from build123d import *

# Parameters (mm, degrees)
F1_DEPTH = 24
F5_R     = 5.08


with BuildPart() as f1:
    # F0 (on Top) → F1 (new body)
    with BuildSketch(Plane.XY):
        with BuildLine():
            Line((-131, 0), (0, 0))
            Line((0, 0), (0, 762))
            Line((0, 762), (-643, 762))
            ThreePointArc((-643, 762), (-996.5533905933, 615.5533905933), (-1143, 262))
            Line((-1143, 262), (-1143, -381))
            Line((-1143, -381), (-381, -381))
            Line((-381, -381), (-381, -250))
            ThreePointArc((-381, -250), (-307.7766952966, -73.2233047034), (-131, 0))
        make_face()
    extrude(amount=F1_DEPTH)

    # F4: sweep along a path in F3
    with BuildLine(Plane(origin=(0, 0, 0), x_dir=(1, 0, 0), z_dir=(0, 0, -1))) as f4_path:
        Line((-381, 381), (-1143, 381))
        Line((-1143, 381), (-1143, -262))
        ThreePointArc((-1143, -262), (-996.5533905933, -615.5533905933), (-643, -762))
        Line((-643, -762), (0, -762))
        Line((0, -762), (0, 0))
        Line((0, 0), (-131, 0))
        ThreePointArc((-131, 0), (-307.7766952966, 73.2233047034), (-381, 250))
        Line((-381, 250), (-381, 381))
    # F2 (on face) → F4 (sweep, cut)
    with BuildSketch(Plane.YZ):
        Polygon((762, 0), (762, 14), (712, 0), align=None)
    sweep(path=f4_path.line, transition=Transition.RIGHT, mode=Mode.SUBTRACT)

    # F5
    f5_edges = [f1.edges().sort_by_distance(p)[0] for p in [
        (0, 762, 19),
        (0, 0, 19),
        (-381, -381, 19),
        (-1143, -381, 19),
    ]]
    fillet(f5_edges, radius=F5_R)


solid = f1.part
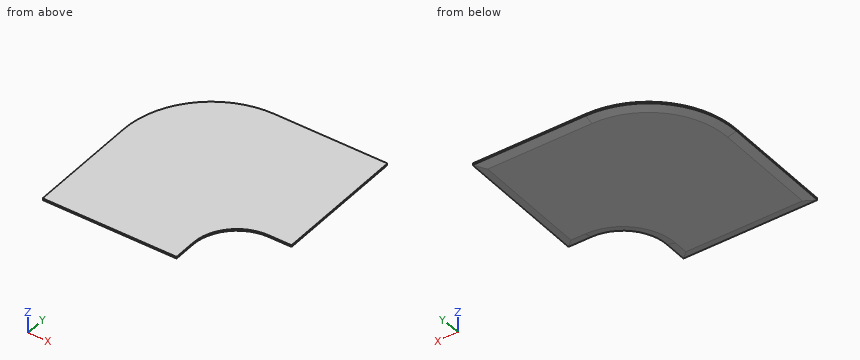
Input: part model. Units: mm. Frame: model coordinates. Coordinates: 2 decimals unless noted, no trailing zeros. Loops run counter-clockwise (first coordinate to the right, second up) from the corner with the lowest first, then second, coordinate; pieces in that order, holes last.
(1) Section B-B on y = 218.5. Return the cut outline in (x, z).
(2) Section A-A on z = 18.25. Return the cut outline in (x, y).
(3) Material intervals for probe 1 along Y at (x, z) = (-71, 20); probe 2 along Y at (x, z) = (-722, 18.25), sorted ascending.
(4) First-contact query: pin 1 Ø1 at (x, y) = (-285, -53.5) entering from -Z; pin 2 Ø5 at (y, z) = (-319, 19) entering from +X; pin 3 Ø5 at (x, z) = (-77.5, 17) entering from -Y. Flat tips, straight axial feed; report the tip coordinate or a pass-through.
(5) Section C-C on x = -542. Return the cut outline in (y, z).
Data:
1. outline: (-1143, 14) - (-1093, 0) - (-50, 0) - (0, 14) - (0, 24) - (-1143, 24) - close
2. outline: (-1143, -375.92) arc R5.08 ccw to (-1137.92, -381) - (-386.08, -381) arc R5.08 ccw to (-381, -375.92) - (-381, -250) arc R250 cw to (-131, 0) - (-5.08, 0) arc R5.08 ccw to (0, 5.08) - (0, 756.92) arc R5.08 ccw to (-5.08, 762) - (-643, 762) arc R500 ccw to (-1143, 262) - close
3. probe 1: y = 0 to 762
3. probe 2: y = -381 to 755.72
4. pin 1: stops at z = 13.96
4. pin 2: stops at x = -381
4. pin 3: stops at y = 0
5. outline: (-381, 14) - (-331, 0) - (712, 0) - (762, 14) - (762, 24) - (-381, 24) - close
